Part model, mm, in its own coordinate system. Face numbers are marked on the shaded views. Give positions to 0.01 mm unless a question says otherwise; leave off trailing zeros. Order: outer loops, then holes, each group sorted by start corner. A loop starts at its lowest first (then second) coordinate and runs counter-clockwise, first axis right, second up. Notation, with made-up numbers: (-32.5, 4.5) - (7.5, 4.5) arc R19 ccw to (7.5, 15.5) - close; hole circle Ø7 at (-11, 76.25). An arc over 180 degrees is marked (long way). One line per item, written item: value.
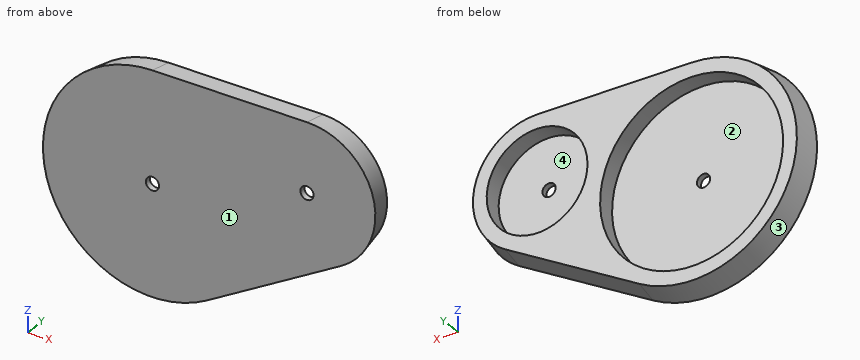
```python
from build123d import *

# Parameters (mm, degrees)
BOSS_EXTRUDE1_DEPTH = 4
BOSS_EXTRUDE1_DRAFT = 10
CUT_EXTRUDE2_START  = 4
SKETCH1_5_R         = 1.1
CUT_EXTRUDE2_DEPTH  = 4
CUT_EXTRUDE3_START  = 4
SKETCH1_6_R         = 15.25
SKETCH1_6_R_2       = 1.1
SKETCH1_6_R_3       = 8.4
CUT_EXTRUDE3_DEPTH  = 3


with BuildPart() as part:
    # Sketch1 → Boss-Extrude1 (with draft: the straight prism first)
    with BuildSketch(Plane(origin=(0, 0, 0), x_dir=(1, 0, 0), z_dir=(0, 1, 0))):
        with BuildLine():
            ThreePointArc((9.066590645, 15.838542675), (-17.636835088, 4.690900563), (0, -18.25))
            Line((0, -18.25), (25.754611238, -18.25))
            ThreePointArc((25.754611238, -18.25), (36.771593155, -9.780206379), (31.418125394, 3.043665013))
            Line((31.418125394, 3.043665013), (9.066590645, 15.838542675))
        make_face()
    extrude(amount=BOSS_EXTRUDE1_DEPTH)
    # Boss-Extrude1: the draft: its side faces are tilted about the plane it starts from
    boss_extrude1_sides = [part.faces().sort_by_distance(p)[0] for p in [
        (-17.636835088, 2, -4.690900563),
        (12.877305619, 2, 18.25),
        (36.771593155, 2, 9.780206379),
        (20.24235802, 2, -9.441103844),
    ]]
    draft(boss_extrude1_sides, Plane(origin=(0, 0, 0), x_dir=(1, 0, 0), z_dir=(0, 1, 0)), BOSS_EXTRUDE1_DRAFT)

    # Sketch1<5> → Cut-Extrude2 (cut)
    with BuildSketch(Plane(origin=(0, 0, 0), x_dir=(1, 0, 0), z_dir=(0, 1, 0)).offset(CUT_EXTRUDE2_START)):
        with Locations(Location((0, 0, 0), (0, 0, 270))):
            Circle(SKETCH1_5_R)
        with Locations(Location((25.754611238, -6.85, 0), (0, 0, 270))):
            Circle(SKETCH1_5_R)
    extrude(amount=-CUT_EXTRUDE2_DEPTH, mode=Mode.SUBTRACT)

    # Sketch1<6> → Cut-Extrude3 (cut)
    # profile 1 of 2: a face of its own
    with BuildSketch(Plane(origin=(0, 0, 0), x_dir=(1, 0, 0), z_dir=(0, 1, 0)).offset(CUT_EXTRUDE3_START)):
        with Locations(Location((0, 0, 0), (0, 0, 270))):
            Circle(SKETCH1_6_R)
        with Locations(Location((0, 0, 0), (0, 0, 270))):
            Circle(SKETCH1_6_R_2, mode=Mode.SUBTRACT)
    # profile 2 of 2: a face of its own
    with BuildSketch(Plane(origin=(0, 0, 0), x_dir=(1, 0, 0), z_dir=(0, 1, 0)).offset(CUT_EXTRUDE3_START)):
        with Locations(Location((25.754611238, -6.85, 0), (0, 0, 270))):
            Circle(SKETCH1_6_R_3)
        with Locations(Location((25.754611238, -6.85, 0), (0, 0, 270))):
            Circle(SKETCH1_6_R_2, mode=Mode.SUBTRACT)
    extrude(amount=-CUT_EXTRUDE3_DEPTH, mode=Mode.SUBTRACT)


solid = part.part
```
1) Drop flat-ended pins along their axis: P1, Ø1.5, axis at x = -9, y = 2.5, coming from the +Z side; P2, Ø9, axis at x = -6.5, z = -3.5, coming from the +Y side. Give the stop position or say it passes through.
Answer:
P1: stops at z = 15.81
P2: stops at y = 1
2) Wall check: line 1 along X through (y, z) = (3.3, 0); line 2 along X through (y, z) = (2.7, 12); line 3 along Z through (x, y) = (-5, 2.85). Give the ranges that are in metal, low to high. Write a range as [from, to].
Answer:
line 1: x = [-17.67, -15.25], [15.25, 20.89], [30.62, 34.13]
line 2: x = [-13.11, -9.41], [9.41, 19.12], [32.39, 35.39]
line 3: z = [-17.03, -14.41], [14.41, 17.03]
3) Two-plate mould, pull along X, no slides. Class the marked faces 1, 2, 3 and 4: pulls with the +X half, pulls with the -X half, needs draft (parallel to the pull), parting line crosses it, or undercut.
Answer:
face 1: needs draft
face 2: undercut
face 3: parting line crosses it
face 4: undercut
4) Slice it at B-B on x = 11. Write the cut outline in (y, z), then the cut area to 3 significant figures.
Answer:
outline: (0, -14.73) - (4, -13.92) - (4, -10.56) - (1, -10.56) - (1, 10.56) - (4, 10.56) - (4, 17.54) - (0, 18.25) - close
area: 65.5 mm2
5) Slice it at A-A on y = 2.65. Write the cut outline in (x, z), then the cut area to 3 significant figures.
Answer:
outline: (0, 17.78) arc R17.78 ccw (long way) to (8.83, -15.43) - (31.19, -2.64) arc R10.93 ccw to (25.75, 17.78) - close; hole circle Ø30.5 at (0, 0); hole circle Ø16.8 at (25.75, 6.85)
area: 523 mm2
